Design review of the part built by this model. Coordinates are the model's own, in mm. Coordinates: 2 decimals unless noted, no trailing zeros. Order: outer loops, then holes, each group sorted by start corner. A loop starts at its lowest first (then second) coordinate and runs counter-clockwise, first axis right, second up. Notation, with made-up numbers: M 25,-25 L 45,-25 A30 ccw 45,10 Z; hole C 79,-4.75 d6. An arc over 180 degrees is marked long. Answer as a JSON object with one key per item and string values.
from build123d import *

# Parameters (mm, degrees)
F0_W     = 25.4
F0_H     = 25.4
F1_DEPTH = 25.4
F2_R     = 4.7625
F3_DEPTH = 64.516
F4_R     = 3.175
F5_DEPTH = 53.594


with BuildPart() as f1:
    # F0 (on Front) → F1 (new body)
    with BuildSketch(Plane.XZ):
        Rectangle(F0_W, F0_H)
    extrude(amount=F1_DEPTH)

    # F2 (on face) → F3 (cut)
    with BuildSketch(Plane.XZ.offset(25.4)):
        Circle(F2_R)
    extrude(amount=-F3_DEPTH, mode=Mode.SUBTRACT)

    # F4 (on face) → F5 (cut)
    with BuildSketch(Plane(origin=(-12.7, 0, 0), x_dir=(0, -1, 0), z_dir=(-1, 0, 0))):
        with Locations((12.440579, 0)):
            Circle(F4_R)
    extrude(amount=-F5_DEPTH, mode=Mode.SUBTRACT)


solid = f1.part
1) To check wall thickness, follow L1, parallel to Z at x = 0, y = -14.75; L2, parallel to Y at x = -9.25, z = 0. State the ranges of each line that lie inside material, in increasing order.
Taken from the geometry:
{"L1": "z = -12.7 to -4.76, 4.76 to 12.7", "L2": "y = -25.4 to -15.62, -9.27 to 0"}
2) Add section A-A (z = 0). State the section outline as (x, y) points.
Taken from the geometry:
{"outline": "M -12.7,-25.4 L -4.76,-25.4 L -4.76,-15.62 L -12.7,-15.62 Z; M -12.7,-9.27 L -4.76,-9.27 L -4.76,0 L -12.7,0 Z; M 4.76,-25.4 L 12.7,-25.4 L 12.7,-15.62 L 4.76,-15.62 Z; M 4.76,-9.27 L 12.7,-9.27 L 12.7,0 L 4.76,0 Z"}
3) Mouldability with a two-part tool opening along Z and no side actions: class faces 1 (the flat face through (12.7, -15, 3)), 2 (the cylindrical face through (8.06, -15.47, 0.95)), 3 (the flat face through (0, -13, -12.7)) as released by +Z, released by -Z, zero draft, split by the parting line, or undercut.
Taken from the geometry:
{"face 1": "zero draft", "face 2": "undercut", "face 3": "released by -Z"}
4) Add section D-D (y = -14.75). State the section outline as (x, z) points (1 decimal), and give its area (3 significant figures).
Taken from the geometry:
{"outline": "M -12.7,-12.7 L 12.7,-12.7 L 12.7,-2.2 L 4.2,-2.2 A4.8 cw -4.2,-2.2 L -12.7,-2.2 Z; M -12.7,2.2 L -4.2,2.2 A4.8 cw 4.2,2.2 L 12.7,2.2 L 12.7,12.7 L -12.7,12.7 Z", "area": "503 mm2"}
5) Insertion check: pin 1 Ø10 at (x, z) = (4, -5.5) entering from +Y; pin 2 Ø5.5 at (y, z) = (-12.44, 0) entering from -X. Each pin has a flat end and moves straight along its axis. Give the tip position at first contact, or say it passes through.
Taken from the geometry:
{"pin 1": "stops at y = 0", "pin 2": "passes through"}
6) Add section B-B (x = 1.5). State the section outline as (y, z) points.
Taken from the geometry:
{"outline": "M -25.4,-12.7 L 0,-12.7 L 0,-4.52 L -25.4,-4.52 Z; M -25.4,4.52 L 0,4.52 L 0,12.7 L -25.4,12.7 Z"}
7) Add section C-C (x = 10.25). State the section outline as (y, z) points (3 decimals), and give its area (3 significant figures).
Taken from the geometry:
{"outline": "M -25.4,-12.7 L 0,-12.7 L 0,12.7 L -25.4,12.7 Z; hole C -12.441,0 d6.35", "area": "613 mm2"}
